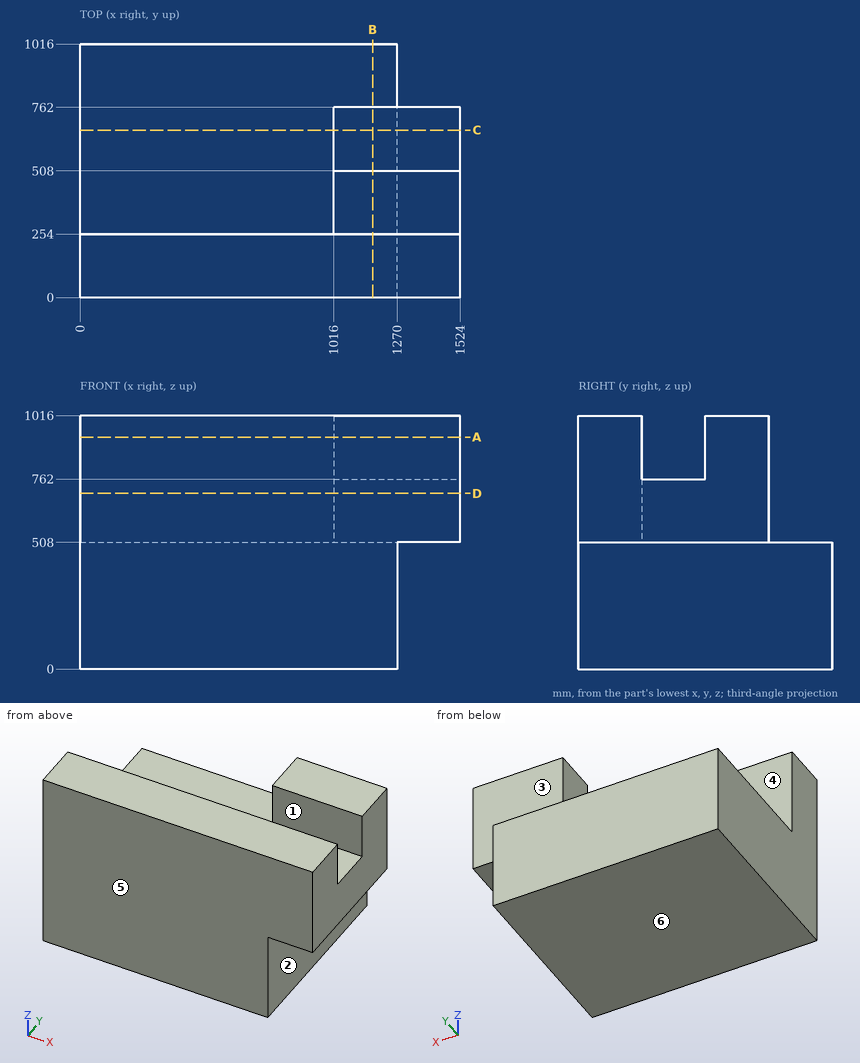
Print and shaded views of the part. All mm, measured from the part's lowest x, y and z. A direction names the side the tool comes from. Coordinates: 2 decimals unless noted, no trailing zeros. Loops run counter-clockwise (first coordinate to the right, second up) from the corner with the lowest first, then second, coordinate; pieces in that order, holes last. Notation, with made-up numbers: (-16, 33) -> (18, 33) arc R29 cw to (18, 55) -> close; hole circle Ø6 at (41.25, 78). An arc over 180 degrees is marked (long way). Use one line per item in the form item = value. Start each with the question number.
(1) Pull direction Y, two halves, no side cores. Call the marked faces 4, 5 and 6: pulls with the +Y half, pulls with the -Y half, needs draft (parallel to the pull), parting line crosses it, or undercut.
(2) Probe probe 1 along Z at (x, y) = (462, 838.5); probe 2 along Y at (x, z) = (92.5, 521); probe 3 along X at (y, z) = (205.5, 450.5). List the from-to ranges inside material, lowest first. Write a range as from..to.
(3) Flat gauge pins, fed straight in: pin 1 (3 mm diameter, centred on x = 530.5, y = 164, fed in from -Z); pin 2 (5 mm diameter, centred on y = 668.5, z = 904, fed in from -X); pin 3 (1.5 mm diameter, centred on x = 688.5, y = 430.5, fed in from +Z). Where does each tip first touch, or does it go through?
(4) Cut at D-D on z = 704. Give the cut face in (x, y), and give its area (3 significant figures).
(5) Cut at C-C on y = 671. Give the cut face in (x, z), and give its area (3 significant figures).
(6) Tool access for the marked faces 1, 2 and 3: list every direction of +Z, -Z, +X, -X, +Y, -Y with a clear straight run to the whole face (end or side of a thin tool).
(7) Cut at B-B on x = 1172. Give the cut face in (y, z).
(8) Cut at A-A on z = 929.5. Give the cut face in (x, y), and give its area (3 significant figures).
Values:
q1.face_4 = undercut
q1.face_5 = pulls with the -Y half
q1.face_6 = needs draft
q2.probe_1 = 0..508
q2.probe_2 = 0..254
q2.probe_3 = 0..1270
q3.pin_1 = 0
q3.pin_2 = 1016
q3.pin_3 = 508
q4.outline = (0, 0) -> (1524, 0) -> (1524, 762) -> (1016, 762) -> (1016, 254) -> (0, 254) -> close
q4.area = 645,000 mm2
q5.outline = (0, 0) -> (1270, 0) -> (1270, 508) -> (1524, 508) -> (1524, 1016) -> (1016, 1016) -> (1016, 508) -> (0, 508) -> close
q5.area = 903,000 mm2
q6.face_1 = +Z, +X, -X
q6.face_2 = -Z, +X, +Y, -Y
q6.face_3 = +Z, +X, -X, +Y
q7.outline = (0, 0) -> (1016, 0) -> (1016, 508) -> (762, 508) -> (762, 1016) -> (508, 1016) -> (508, 762) -> (254, 762) -> (254, 1016) -> (0, 1016) -> close
q8.outline = (0, 0) -> (1524, 0) -> (1524, 254) -> (0, 254) -> close; (1016, 508) -> (1524, 508) -> (1524, 762) -> (1016, 762) -> close
q8.area = 516,000 mm2
